Read the model definition and answer for the solid it produces. Units are mm, in the model's axes. A direction names the side the tool comes from. Coordinates: 2 decimals unless noted, no trailing zeros. Write each loop counter-clockwise with the first axis right and the second up, starting at its lowest first coordinate (ties: lowest second). Pieces come first, ordered by that corner, then holes.
from build123d import *

# Parameters (mm, degrees)
SKETCH_1_W = 3.5
SKETCH_1_H = 7.5


with BuildPart() as part:
    # 草图1 → 旋转1 (revolve)
    with BuildSketch(Plane(origin=(0, 0, 0), x_dir=(0, 0, -1), z_dir=(1, 0, 0)), mode=Mode.PRIVATE) as revolve_1_sk:
        with Locations((3.75, -3.75)):
            Rectangle(SKETCH_1_W, SKETCH_1_H)
        Polygon((5.5, -7.5), (2, -7.5), (2, -8.9), (3.1, -8.9), (3.1, -11.5), (11, -11.5), (11, -7.5), align=None)
    revolve(revolve_1_sk.sketch.rotate(Axis((0, 0, 0), (0, -1, 0)), 180), axis=Axis((0, 0, 0), (0, -1, 0)))


solid = part.part
Item 1: Given pin 1 (1 mm diameter, centred on y = -6, z = -3, fed in from -X); pin 2 (3 mm diameter, centred on x = 7.5, z = 5.5, fed in from +Y); pin 3 (5 mm diameter, centred on x = -1, y = -3, fed in from +Z), each flat-ended and moving along its own axis, determine where each tip first touches the part or whether it passes through.
Item 2: The part is cut by section A-A (z = 0). Give the vertices of the cut face in (x, y).
Item 3: The part is cut by section B-B (x = 0). Give the vertices of the cut face in (y, z), and give its area (3 significant figures).
Item 4: The part is cut by section C-C (y = -4). Give the vertices of the cut face in (x, z), and give its area (3 significant figures).
Item 5: Find the intervals of material crossed by probe 1 along X at (y, z) = (-1.75, 0); probe 2 along X at (y, z) = (-10.75, 0); probe 3 along Y at (x, z) = (2.25, -9), in increasing order.
Item 6: Determine the mould class of faces 4 (the cylindrical face through (5.37, -3.7, -1.19)), 5 (the cylindrical face through (2, -5, 0)), 6 (the flat face through (2.4, 0, 0.1)) for opening direction X: +X half, -X half, draft (parallel to the pull), parting line (faces both ways), or undercut.
Item 7: For faces 1 (the flat face through (2.3, -11.5, -2.3)), 2 (the cylindrical face through (-0.931, -10.218, 2.957)), 3 (the flat face through (-3, -7.5, -5)), determine the directions among +Z, -Z, +X, -X, +Y, -Y from which every point of the face is accessible in a straight line to the end or side of a thin tool.
Item 8: The part is cut by section D-D (x = 4). Give the vertices of the cut face in (y, z), and give its area (3 significant figures).
Answer:
1. pin 1: stops at x = -4.9
1. pin 2: stops at y = -7.5
1. pin 3: stops at z = 5.5
2. outline: (-11, -11.5) - (-3.1, -11.5) - (-3.1, -8.9) - (-2, -8.9) - (-2, 0) - (-5.5, 0) - (-5.5, -7.5) - (-11, -7.5) - close; (2, -8.9) - (3.1, -8.9) - (3.1, -11.5) - (11, -11.5) - (11, -7.5) - (5.5, -7.5) - (5.5, 0) - (2, 0) - close
3. outline: (-11.5, -11) - (-7.5, -11) - (-7.5, -5.5) - (0, -5.5) - (0, -2) - (-8.9, -2) - (-8.9, -3.1) - (-11.5, -3.1) - close; (-11.5, 3.1) - (-8.9, 3.1) - (-8.9, 2) - (0, 2) - (0, 5.5) - (-7.5, 5.5) - (-7.5, 11) - (-11.5, 11) - close
3. area: 119 mm2
4. outline: circle Ø11 at (0, 0); hole circle Ø4 at (0, 0)
4. area: 82.5 mm2
5. probe 1: x = -5.5 to -2, 2 to 5.5
5. probe 2: x = -11 to -3.1, 3.1 to 11
5. probe 3: y = -11.5 to -7.5
6. face 4: parting line
6. face 5: undercut
6. face 6: draft
7. face 1: +Z, -Z, +X, -X, -Y
7. face 2: -Y
7. face 3: +Y
8. outline: (-11.5, -10.25) - (-7.5, -10.25) - (-7.5, -3.77) - (0, -3.77) - (0, 3.77) - (-7.5, 3.77) - (-7.5, 10.25) - (-11.5, 10.25) - close
8. area: 139 mm2
